from build123d import *

# Parameters (mm, degrees)
F0_W     = 215
F0_H     = 145
F1_DEPTH = 4
F2_R     = 1.5
F3_DEPTH = 4.001
F4_W     = 50
F4_H     = 70
F5_DEPTH = 4.001
F6_R     = 1.6
F6_R_2   = 1
F7_DEPTH = 4.001


with BuildPart() as f1:
    # F0 (on Top) → F1 (new body)
    with BuildSketch(Plane.XY):
        Rectangle(F0_W, F0_H)
    extrude(amount=F1_DEPTH)

    # F2 (on face) → F3 (cut, through all)
    with BuildSketch(Plane.XY.offset(4)):
        with Locations((-94.5, -63.5)):
            Circle(F2_R)
        with Locations((85.5, -63.5)):
            Circle(F2_R)
    extrude(amount=-F3_DEPTH, mode=Mode.SUBTRACT)

    # F4 (on face) → F5 (cut, through all)
    with BuildSketch(Plane.XY.offset(4)):
        with Locations((82.5, 37.5)):
            Rectangle(F4_W, F4_H)
    extrude(amount=-F5_DEPTH, mode=Mode.SUBTRACT)

    # F6 (on face) → F7 (cut, through all)
    with BuildSketch(Plane.XY.offset(4)):
        with Locations((-101.5, 66.5)):
            Circle(F6_R)
        with Locations((-77.5, 66.5)):
            Circle(F6_R)
        with Locations((-77.5, 42.5)):
            Circle(F6_R)
        with Locations((-101.5, 42.5)):
            Circle(F6_R)
        with Locations((-101.5, 35.5)):
            Circle(F6_R)
        with Locations((-77.5, 35.5)):
            Circle(F6_R)
        with Locations((-77.5, 11.5)):
            Circle(F6_R)
        with Locations((-101.5, 11.5)):
            Circle(F6_R)
        with Locations((101.5, -21.5)):
            Circle(F6_R_2)
        with Locations((84.5, -21.5)):
            Circle(F6_R_2)
        with Locations((101.5, -45.5)):
            Circle(F6_R_2)
        with Locations((84.5, -45.5)):
            Circle(F6_R_2)
        with Locations((77.5, -21.5)):
            Circle(F6_R_2)
        with Locations((60.5, -21.5)):
            Circle(F6_R_2)
        with Locations((77.5, -45.5)):
            Circle(F6_R_2)
        with Locations((60.5, -45.5)):
            Circle(F6_R_2)
        with Locations((53.5, -21.5)):
            Circle(F6_R_2)
        with Locations((36.5, -21.5)):
            Circle(F6_R_2)
        with Locations((53.5, -45.5)):
            Circle(F6_R_2)
        with Locations((36.5, -45.5)):
            Circle(F6_R_2)
        with Locations((43.41, 58.41)):
            Circle(F6_R)
        with Locations((11.59, 58.41)):
            Circle(F6_R)
        with Locations((5, 65)):
            Circle(F6_R)
        with Locations((50, 65)):
            Circle(F6_R)
        with Locations((50, 20)):
            Circle(F6_R)
        with Locations((43.41, 26.59)):
            Circle(F6_R)
        with Locations((11.59, 26.59)):
            Circle(F6_R)
        with Locations((5, 20)):
            Circle(F6_R)
        with Locations((3.5, -14.5)):
            Circle(F6_R_2)
        with Locations((20.5, -14.5)):
            Circle(F6_R_2)
        with Locations((3.5, -56.5)):
            Circle(F6_R_2)
        with Locations((20.5, -56.5)):
            Circle(F6_R_2)
        with Locations((-82.862776, -57.2)):
            Circle(F6_R_2)
        with Locations((-34.662776, -58.5)):
            Circle(F6_R_2)
        with Locations((-39.762776, -6.4)):
            Circle(F6_R_2)
        with Locations((-67.662776, -6.4)):
            Circle(F6_R_2)
    extrude(amount=-F7_DEPTH, mode=Mode.SUBTRACT)


solid = f1.part
Verification items for the finished model (mm, model axes). A direction names the side the tool comes from. Give positions to 0.01 mm unless a question says otherwise; leave off trailing zeros. Loops run counter-clockwise (first coordinate to the right, second up) from the corner with the lowest first, then second, coordinate; pieces in that order, holes last. Notation, with made-up numbers: (69, 15) - (103, 15) arc R24 cw to (103, 50) - close; hole circle Ø4 at (56, 12.25). An arc over 180 degrees is marked (long way). Write each question's results on one line, items separated by ' | '.
1) Depth check by flat-ended pin: P1, Ø3, axis at x = 36.5, y = -21.5, coming from the -Z side; P2, Ø2, axis at y = 36.5, z = 1.5, coming from the +X side. Enter the tip coordinate at first touch or a pass-through.
Solution:
P1: z = 0 | P2: x = 57.5
2) Sectioned sample at A-A on x = 72.5. Record the boundary of the cut face in (y, z).
Solution:
outline: (-72.5, 0) - (2.5, 0) - (2.5, 4) - (-72.5, 4) - close
3) Tool access check on faces 1 (the flat face through (82, 2.5, 2)), 2 (the flat face through (-2, 1, 0)). Record the directions out of +Z, -Z, +X, -X, +Y, -Y that give a thin tool (end or side, any length) a straight path to the whole face; none if there is none.
Solution:
face 1: +Z, -Z, +X, +Y | face 2: -Z, +X, -X, +Y, -Y
4) Material ranges on L1, parallel to Y at x = 11.59, z = 1.25; L2, parallel to Y at x = 50, z = 1; L3, parallel to Y at x = -77.5, z = 2.15, recorded low to high. Write a range as from..to.
Solution:
L1: -72.5..24.99, 28.19..56.81, 60.01..72.5 | L2: -72.5..18.4, 21.6..63.4, 66.6..72.5 | L3: -72.5..9.9, 13.1..33.9, 37.1..40.9, 44.1..64.9, 68.1..72.5
